The model under review builds one solid part; all positions refer to its coordinate system, in mm. Face numbers are marked on the shaded views. A direction names the side the tool comes from. Round coordinates to 2 decimals unless told otherwise and drop trailing zeros. Order: outer loops, then holes, each group sorted by start corner. A loop starts at its lowest first (then second) coordinate and runs counter-clockwise, first axis right, second up. Notation, with made-up numbers: M -26.5,6 L 24.5,6 A22 ccw 24.5,12 Z; hole C 22,36.25 d3. An arc over 180 degrees is marked long. Use a Markdown table: item, result. Add a question column.
1. Consider section A-A on x = -15. State the section outline as (y, z) points, then the cut area to 3 significant figures.
2. To check wall thickness, follow probe 1 along X at (y, z) = (1, 1); probe 2 along X at (y, z) = (-4, 0.25); probe 3 along Y at (x, z) = (-7, -2). State the ranges of each line that lie inside material, in increasing order.
3. For the marked faces 1, 2 and 3, list the 3-axis set-ups (+Z, -Z, +X, -X, +Y, -Y) from which the entire face can be reached by the end or side of a thin tool; tool diameter is ignored.
4. The part is to be moulded in two halves that separate along Z. For the marked faces 4, 5 and 6, say which applies: +Z half, -Z half, draft (parallel to the pull), parting line (faces both ways), or undercut.
5. Insertion check: P1, Ø3, axis at x = -9, z = -2, coming from the -Y side; P2, Ø4, axis at x = -14, y = -2.5, coming from the -Z side; P3, Ø1.5, axis at y = -0.5, z = 0.5, coming from the -X side. Each pin has a flat end and moves straight along its axis. Give the tip position at first contact, or say it passes through.
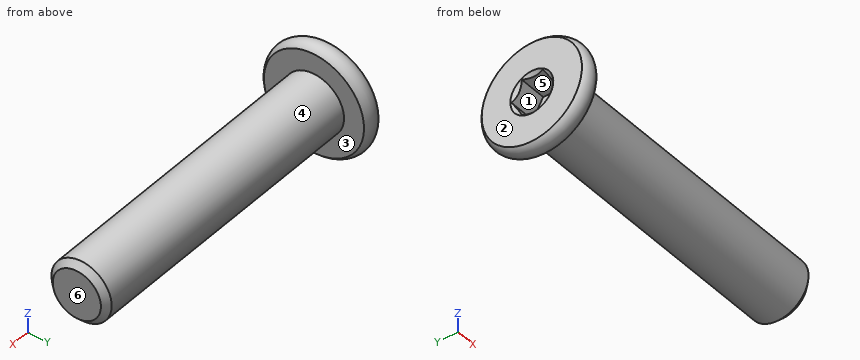
from build123d import *

# Parameters (mm, degrees)
SKETCH2_R           = 2.5
BOSS_EXTRUDE1_DEPTH = 25
CHAMFER1_SIZE       = 0.5
CUT_EXTRUDE1_DEPTH  = 2.3
SKETCH8_R           = 1.782050808
CUT_EXTRUDE2_DEPTH  = 1
CUT_EXTRUDE2_TAPER  = 45


with BuildPart() as part:
    # Sketch2 → Boss-Extrude1 (new body)
    with BuildSketch(Plane(origin=(0, 0, 0), x_dir=(0, 0, -1), z_dir=(1, 0, 0))):
        Circle(SKETCH2_R)
    extrude(amount=-BOSS_EXTRUDE1_DEPTH)

    # Chamfer1
    chamfer1_edges = [part.edges().sort_by_distance(p)[0] for p in [
        (0, 0, 2.5),
    ]]
    chamfer(chamfer1_edges, length=CHAMFER1_SIZE)

    # Sketch6 → Revolve1 (revolve)
    with BuildSketch(Plane.XY):
        with BuildLine():
            Line((-26.5, 0), (-26.5, 4.161437828))
            ThreePointArc((-26.5, 4.161437828), (-25.75, 4.5), (-25, 4.161437828))
            Line((-25, 4.161437828), (-25, 0))
            Line((-25, 0), (-26.5, 0))
        make_face()
    revolve(axis=Axis((-25, 0, 0), (1, 0, 0)))

    # Sketch7 → Cut-Extrude1 (cut)
    with BuildSketch(Plane.ZY.offset(26.5)):
        Polygon((0, 1.732050808), (-1.5, 0.866025404), (-1.5, -0.866025404), (0, -1.732050808), (1.5, -0.866025404), (1.5, 0.866025404), align=None)
    extrude(amount=-CUT_EXTRUDE1_DEPTH, mode=Mode.SUBTRACT)

    # Sketch8 → Cut-Extrude2 (cut)
    with BuildSketch(Plane.ZY.offset(26.5)):
        Circle(SKETCH8_R)
    extrude(amount=-CUT_EXTRUDE2_DEPTH, taper=CUT_EXTRUDE2_TAPER, mode=Mode.SUBTRACT)


solid = part.part
Answer block:
| question | item | result |
|---|---|---|
| 1 | outline | C 0,0 d5 |
| 1 | area | 19.6 mm^2 |
| 2 | probe 1 | -24.2 to 0 |
| 2 | probe 2 | -26.5 to -25 |
| 2 | probe 3 | -1.5 to 1.5 |
| 3 | face 1 | -X |
| 3 | face 2 | +Z, -Z, -X, +Y, -Y |
| 3 | face 3 | +X |
| 4 | face 4 | parting line |
| 4 | face 5 | undercut |
| 4 | face 6 | draft |
| 5 | P1 | y = -2.45 |
| 5 | P2 | z = -2.45 |
| 5 | P3 | x = -24.2 |
